Source: CAD feature listing. Evaluate the final solid. Frame: model axes, mm. A direction names the side the tool comes from. Round coordinates to 2 decimals unless told otherwise and drop trailing zeros. Order: outer loops, then holes, each group sorted by start corner. A loop starts at its lowest first (then second) coordinate and runs counter-clockwise, first axis right, second up. Notation, with made-up numbers: (10.25, 27.5) - (36.25, 27.5) arc R8 cw to (36.25, 42.5) - close; hole circle Ø3 at (36.25, 23.5). An arc over 180 degrees is marked (long way). Put each result on its own line as item: value. Start each with the question number.
1) Section A-A on x = 67.5. Output: boundary loops of the cut face in (y, z).
2) Line query: probe 1 along Y at (x, z) = (39.5, 7.5); probe 2 along X at (y, z) = (28.5, 11.5); probe 3 along X at (y, z) = (12, 16.5). Output: solid intervals per line, ascending. Write a range as [from, to].
3) Access query for faces 1 (the face through (-37.266, 51.903, 8.034)), 2 (the face through (-15.39, 55.1, 9.46)). Directions: +Z, -Z, +X, -X, +Y, -Y. A direction counts if a zero-diameter tool reaches every point of the face in a straight line with its end or side. Return the directions, or none.
4) Contact query for flat-ended pins moving along their axis: P1, Ø1.5, axis at y = 35.5, z = 10.5, coming from the -X side; P2, Ø1.5, axis at x = -4.5, y = 54.5, coming from the -Z side; P3, Ø1.5, axis at x = 4.5, z = 19.5, coming from the +Y side. Output: stop coordinate, or through.
5) Section B-B on y = 18.5. Output: boundary loops of the cut face in (x, z), then the cut area to 3 significant figures.
6) Mould query, pull axis Z, two halves, no side actions, for faces 3 (the face through (-13.8, 55.1, 12.62)), 4 (the face through (57, 29, 23)), 5 (the face through (53, 4.081, 11)). Classes: +Z half, -Z half, draft (parallel to the pull), parting line (faces both ways), or undercut.
Autodesk Inventor part; units mm, degrees
ref_plane "Płaszczyzna konstrukcyjna1" through (0, 0, 15) normal (0, 0, 1) x (1, 0, 0)
ref_plane "YZ Plane" through (0, 0, 0) normal (1, 0, 0) x (0, 1, 0)
ref_plane "XZ Plane" through (0, 0, 0) normal (0, 1, 0) x (-1, 0, 0)
sketch "Szkic1" plane through (0, 0, 0) normal (0, 0, 1) x (1, 0, 0)
  line L0 (-17.4978, 4.0814) -> (126.0022, 4.0814)
  line L1 (126.0022, 4.0814) -> (126.0022, 54.0814)
  line L2 (126.0022, 54.0814) -> (-17.4978, 54.0814)
  line L3 (-17.4978, 54.0814) -> (-17.4978, 4.0814)
  point P0 (0, 0)
  dimension "d0" = 143.5
  dimension "d1" = 50
extrude "Wyciągnięcie proste1" add sketch "Szkic1" along normal blind 23
fillet "Zaokrąglenie1" radius 9 2 edges at (-17.4978, 29.0814, 23) (-17.4978, 29.0814, 0)
fillet "Zaokrąglenie2" radius 2 2 edges at (126.0022, 4.0814, 11.5) (126.0022, 54.0814, 11.5)
fillet "Zaokrąglenie3" radius 1 16 edges at (125.4164, 4.6672, 23) (126.0022, 29.0814, 23) (125.4164, 53.4956, 23) (57.7522, 54.0814, 23) (-14.8618, 54.0814, 20.364) (-17.4978, 54.0814, 11.5) (-14.8618, 54.0814, 2.636) (57.7522, 54.0814, 0) (125.4164, 53.4956, 0) (126.0022, 29.0814, 0) (125.4164, 4.6672, 0) (57.7522, 4.0814, 0) (-14.8618, 4.0814, 2.636) (-17.4978, 4.0814, 11.5) (-14.8618, 4.0814, 20.364) (57.7522, 4.0814, 23)
sketch "Szkic2" plane through (0, 0, 23) normal (0, 0, 1) x (1, 0, 0)
  line L0 (2.5572, 48.5476) -> (113.8689, 48.5476) construction
  line L1 (113.8689, 48.5476) -> (113.8689, 11.3084) construction
  line L2 (113.8689, 11.3084) -> (2.5572, 11.3084) construction
  line L3 (2.5572, 11.3084) -> (2.5572, 48.5476) construction
  point P0 (0, 0)
ref_plane "Płaszczyzna konstrukcyjna1" through (0, 0, 15) normal (0, 0, 1) x (1, 0, 0)
sketch "Szkic3" plane through (0, 0, 15) normal (0, 0, 1) x (1, 0, 0)
  line L0 (-16.4978, 54.0814) -> (-8.4978, 54.0814)
  line L1 (-17.4978, 53.0814) -> (-17.4978, 5.0814)
  line L2 (-13.4978, 54.0814) -> (-13.4978, 56.0814)
  line L3 (-18.4978, 60.0814) -> (-17.4978, 60.0814)
  arc A0 (-13.4978, 56.0814) -> (-17.4978, 60.0814) centre (-17.4978, 56.0814) ccw
  line L4 (-18.4978, 60.0814) -> (-21.2325, 60.0814)
  line L5 (-24.203, 59.2945) -> (-37.2438, 51.8639)
  arc A1 (-21.2325, 60.0814) -> (-24.203, 59.2945) centre (-21.2325, 54.0814) ccw
  point P0 (0, 0)
  point P1 (-13.4978, 58.0814)
  dimension "d15" = 4
  dimension "d16" = 4
  dimension "d20" = 4
  dimension "d24" = 6
  dimension "d25" = 6
sketch "Szkic4" plane through (-8.4978, 54.0814, 1) normal (0, 1, 0) x (1, 0, 0)
  circle A0 centre (-4.9887, -14.0009) radius 2.4
  point P0 (8.4978, 1)
  dimension "d21" = 4.8
sweep "Przeciągnięcie1" add profiles "Szkic4" path "Szkic3" path curves L2 A0 L3 L4 A1 L5
pattern_linear "Szyk prostokątny1" count 2 spacing 7 along (0, 0, -1) of "Przeciągnięcie1"
decal "Pokrycie bitmapą1"
properties part number "COTS_ZIPPY_Li-Po_Battery_5000mAh_3S"
Answer sheet:
1. outline: (4.08, 1) arc R1 ccw to (5.08, 0) - (53.08, 0) arc R1 ccw to (54.08, 1) - (54.08, 22) arc R1 ccw to (53.08, 23) - (5.08, 23) arc R1 ccw to (4.08, 22) - close
2. probe 1: [4.08, 54.08]
2. probe 2: [-17.5, 126]
2. probe 3: [-17.14, 126]
3. face 1: +Z, -Z, -X, -Y
3. face 2: none
4. P1: x = -17.5
4. P2: z = 0.26
4. P3: y = 54.08
5. outline: (-17.5, 9) arc R9 ccw to (-8.5, 0) - (125, 0) arc R1 ccw to (126, 1) - (126, 22) arc R1 ccw to (125, 23) - (-8.5, 23) arc R9 ccw to (-17.5, 14) - close
5. area: 3,270 mm^2
6. face 3: undercut
6. face 4: +Z half
6. face 5: draft
